Autodesk Inventor part; units mm, degrees
ref_plane "MSC_PF1" through (0, 0, 0) normal (0, 1, 0) x (-1, 0, 0)
ref_plane "MSC_PT1" through (0, 0, 13.5999) normal (0, 0, -1) x (-1, 0, 0)
ref_plane "YZ Plane" through (0, 0, 0) normal (1, 0, 0) x (0, 1, 0)
sketch "Sketch2" plane through (0, 0, 0) normal (0, 1, 0) x (-1, 0, 0)
  line L0 (0, 13.5999) -> (0, -36.4001)
  line L1 (0, -36.4001) -> (5.125, -36.4001)
  line L2 (6, -35.5251) -> (6, -6.4001)
  line L3 (6, -6.4001) -> (5.35, -5.2742)
  line L4 (5.35, -5.2742) -> (5.35, 13.5999)
  line L5 (5.35, 13.5999) -> (0, 13.5999)
  line L6 (5.125, -36.4001) -> (6, -35.5251)
  line L7 (6, -36.4001) -> (6, -37.6375)
  line L8 (0, -47.885) -> (0, 23.8474)
  dimension "Ds" = 10.7
  dimension "NND" = 12
  dimension "b" = 30
  dimension "d3" = 30
  dimension "d5" = 45
  dimension "PTC" = 1.75
  dimension "NLG" = 50
revolve "Revolution1" add sketch "Sketch2" angle 360 about axis through (0, 0, 13.5999) along (0, 0, -1)
sketch "Sketch3" plane through (0, 0, 13.5999) normal (0, 0, 1) x (1, 0, 0)
  circle A0 centre (0, 0) radius 5.35
  line L0 (0, 9) -> (5.1962, 9)
  line L1 (5.1962, 9) -> (10.3923, 0)
  line L2 (10.3923, 0) -> (0, 0)
  line L3 (0, 0) -> (0, 9)
  line L4 (0, 9) -> (-5.1962, 9)
  line L5 (-5.1962, 9) -> (-10.3923, 0)
  line L6 (0, -9) -> (5.1962, -9)
  line L7 (5.1962, -9) -> (10.3923, 0)
  line L8 (-5.1962, -9) -> (-10.3923, 0)
  line L9 (0, -9) -> (-5.1962, -9)
  dimension "d9" = 60
  dimension "ParS" = 18
  dimension "msp_d11" = 18
extrude "Extrusion1" add sketch "Sketch3" along normal blind 7.5
sketch "Sketch4" plane through (0, 0, 0) normal (0, 1, 0) x (-1, 0, 0)
  line L0 (-9, 21.0999) -> (-10.3923, 21.0999)
  line L1 (-10.3923, 21.0999) -> (-10.3923, 20.2961)
  line L2 (-10.3923, 20.2961) -> (-9, 21.0999)
  line L3 (0, 10.7234) -> (0, 30.8591)
  line L4 (0, 27.9826) -> (0, 27.1787)
  line L5 (-10.3923, 13.5999) -> (-10.3923, 21.0999)
  line L6 (-5.1962, 21.0999) -> (-10.3923, 21.0999)
  dimension "d14" = 30
  dimension "msp_d15" = 18
revolve "Revolution2" cut sketch "Sketch4" angle 360 about axis through (0, 0, 27.9826) along (0, 0, -1)
sketch "Sketch5" plane through (0, 0, 21.0999) normal (0, 0, 1) x (1, 0, 0)
  arc A0 (7.7942, 4.5) -> (0, 9) centre (0, 0) ccw
  circle A1 centre (0, 0) radius 6.75
  dimension "d27" = 13.5
extrude "Extrusion2" cut sketch "Sketch5" against normal blind 1.5
thread "Thread1"
ref_plane "MSC_PF1" through (0, 0, 0) normal (0, 1, 0) x (-1, 0, 0)
ref_plane "MSC_PT1" through (0, 0, 13.5999) normal (0, 0, -1) x (-1, 0, 0)
fillet "Fillet1" radius 0.6 1 edges at (5.35, 0, 13.5999)
equation "\"msp_d11\" = ParS"
equation "\"msp_d15\" = ParS"
equation "\"d27\" = 0.75 * ParS"
equation "\"d28\" = 0.2 * ParK"
equation "\"d30\" = r"
equation "\"msp_d17\" = b"
equation "\"r\" = 0.6"
equation "\"THREADDIA\" = NND"
properties part number "ISO 4015 - M12 x 50" material "Stainless Steel, 440C"
For this review, take the finished solid that the model builds, in its own axes (mm). A direction names the side the tool comes from. Coordinates: 2 decimals unless noted, no trailing zeros. Write each loop counter-clockwise with the first axis right and the second up, starting at its lowest first coordinate (ties: lowest second). Pieces come first, ordered by that corner, then holes.
(1) The part is to be moulded in two halves that separate along Z. For faces 4 (the face through (-1.46, -6.59, 20.36)), 5 (the face through (1.16, 5.223, 3.991)), 6 (the face through (-9.338, -0.023, 20.905)), 7 (the face through (0, 0, -36.4)), say which applies: +Z half, -Z half, draft (parallel to the pull), parting line (faces both ways), or undercut.
(2) For pin 1 Ø8 at (x, z) = (4.5, -11.5) entering from +Y; pin 2 Ø2 at (x, z) = (2, -13) entering from +Y; pin 3 Ø6 at (y, z) = (0.5, -15) entering from -X, all flat-tipped, find the tip position at first contact; note any pin that passes through.
(3) Add section A-A on z = 16. Give the boundary of the cut face in (x, y).
(4) Add section B-B on z = -31. Give the boundary of the cut face in (x, y).
(5) Tool access review of faces 1 (the face through (0, 0, 19.6)), 2 (the face through (0, -9, 17)), 3 (the face through (6, 0, -21)): name each direction out of +Z, -Z, +X, -X, +Y, -Y from which nothing blocks a thin tool from reaching the whole face with its end or side.
(6) Wall thickness on probe 1 along Y at (x, z) = (0, 20.75); probe 2 along Z at (x, y) = (6.25, -0.75); probe 3 along Y at (x, z) = (0.25, -28): over which ranges is each line inside the solid? List them lowest first.
Answer sheet:
1. face 4: draft
1. face 5: undercut
1. face 6: +Z half
1. face 7: -Z half
2. pin 1: stops at y = 5.98
2. pin 2: stops at y = 5.92
2. pin 3: stops at x = -6
3. outline: (-10.39, 0) - (-5.2, -9) - (5.2, -9) - (10.39, 0) - (5.2, 9) - (-5.2, 9) - close
4. outline: circle Ø12 at (0, 0)
5. face 1: +Z
5. face 2: +Z, -Z, +X, -X, -Y
5. face 3: -Z
6. probe 1: y = -9 to -6.75, 6.75 to 9
6. probe 2: z = 13.6 to 19.6
6. probe 3: y = -5.99 to 5.99
